Build history of the part. All positions in model axes, mm. A direction names the side the tool comes from. Coordinates: 2 decimals unless noted, no trailing zeros. Loops run counter-clockwise (first coordinate to the right, second up) from the corner with the lowest first, then second, coordinate; pieces in that order, holes last.
Item 1: Mould opens along X. For faces 1 (the face through (15.7, -17.4, 0)), 2 (the face through (-31.771, -29.148, -33.479)), 3 (the face through (-48.483, -0.7, -33.479)), 4 (the face through (19.435, -14.902, -17.745)) say: released by +X, released by -X, zero draft, split by the parting line, or undercut.
Item 2: 3-axis set-ups, long thin cutter, end or side, ignore diameter. For faces 5 (the face through (22, 19, -32)), 6 (the face through (0, 41.588, -33)): which of +Z, -Z, +X, -X, +Y, -Y reach the whole face in a straight line?
Item 3: Cut at C-C (y = -30.5). List the corners of the cut face in (x, z).
Item 4: Cut at D-D (z = -26.5). List the corners of the cut face in (x, y), and give its area (3 significant figures).
Item 5: Drill centre lines: line 1 along Z through (x, y) = (-36.5, -30.5); line 2 along X through (y, z) = (22, -22.5); line 3 along Y through (x, z) = (-18.5, -30.5). Where is each one in solid material? Low to high.
Item 6: Flat gauge pins, fed straight in: pin 1 (10 mm diameter, centred on y = -14.5, z = -8, fed in from +X); pin 2 (5 mm diameter, centred on y = 4, z = -22, fed in from +X); pin 3 (6 mm diameter, centred on x = 31.5, y = 7, fed in from +Z). Where does each tip first touch, or does it go through?
Item 7: Cut at A-A (x = 0). List the corners of the cut face in (y, z).
Item 8: Cut at B-B (y = 0). List the corners of the cut face in (x, z), and give its area (3 significant figures).
from build123d import *

# Parameters (mm, degrees)
SKETCH3_R          = 1.9
CUT_EXTRUDE1_DEPTH = 4
CIRPATTERN1_COUNT  = 8
SKETCH4_W          = 196.975315964
SKETCH4_H          = 183.175315964
SKETCH4_W_2        = 96.975315964
SKETCH4_H_2        = 83.175315964
CUT_EXTRUDE2_DEPTH = 4


with BuildPart() as part:
    # Sketch2 → Revolve1 (revolve)
    with BuildSketch(Plane(origin=(0, 0, 0), x_dir=(1, 0, 0), z_dir=(0, 1, 0))):
        Polygon((-28.697438418, 35), (-26.25, 0), (-23.25, 0), (-25.697438418, 35), align=None)
        Polygon((-28.487657982, 32), (-28.697438418, 35), (-48.487657982, 35), (-48.487657982, 32), align=None)
    revolve(axis=Axis((0, 0, 0), (0, 0, -1)))

    # Sketch3 → Cut-Extrude1 (cut, through all)
    with BuildSketch(Plane.XY.offset(-32)):
        with Locations((43.487657982, 0)):
            Circle(SKETCH3_R)
    cut_extrude1 = extrude(amount=-CUT_EXTRUDE1_DEPTH, mode=Mode.SUBTRACT)

    # CirPattern1: Cut-Extrude1 ×8 about axis
    cirpattern1_axis = Axis((0, 0, 0), (0, 0, 1))
    for i in range(1, CIRPATTERN1_COUNT):
        add(cut_extrude1.rotate(cirpattern1_axis, i * 360 / CIRPATTERN1_COUNT), mode=Mode.SUBTRACT)

    # Sketch4 → Cut-Extrude2 (cut, through all)
    with BuildSketch(Plane.XY.offset(-32)):
        Rectangle(SKETCH4_W, SKETCH4_H)
        Rectangle(SKETCH4_W_2, SKETCH4_H_2, mode=Mode.SUBTRACT)
    extrude(amount=-CUT_EXTRUDE2_DEPTH, mode=Mode.SUBTRACT)


solid = part.part
Filled sheet:
1. face 1: zero draft
1. face 2: undercut
1. face 3: released by -X
1. face 4: undercut
2. face 5: +Z
2. face 6: +Z, -Z, +X, -X, +Y
3. outline: (-37.69, -35) - (-32.63, -35) - (-32.63, -32) - (-37.69, -32) - close; (-28.87, -35) - (28.87, -35) - (28.87, -32) - (-28.87, -32) - close; (32.63, -35) - (37.69, -35) - (37.69, -32) - (32.63, -32) - close
4. outline: circle Ø56.21 at (0, 0); hole circle Ø50.21 at (0, 0)
4. area: 501 mm2
5. line 1: z = -35 to -32
5. line 2: x = -17.03 to -11.5, 11.5 to 17.03
5. line 3: y = -21.53 to -17.38, 17.38 to 21.53
6. pin 1: stops at x = 25.11
6. pin 2: stops at x = 27.82
6. pin 3: stops at z = -32
7. outline: (-41.59, -35) - (-25.7, -35) - (-23.25, 0) - (-26.25, 0) - (-28.49, -32) - (-41.59, -32) - close; (23.25, 0) - (25.7, -35) - (41.59, -35) - (41.59, -32) - (28.49, -32) - (26.25, 0) - close
8. outline: (-48.49, -35) - (-45.39, -35) - (-45.39, -32) - (-48.49, -32) - close; (-41.59, -35) - (-25.7, -35) - (-23.25, 0) - (-26.25, 0) - (-28.49, -32) - (-41.59, -32) - close; (23.25, 0) - (25.7, -35) - (41.59, -35) - (41.59, -32) - (28.49, -32) - (26.25, 0) - close; (45.39, -35) - (48.49, -35) - (48.49, -32) - (45.39, -32) - close
8. area: 307 mm2
